```python
from build123d import *

# Parameters (mm, degrees)
SKETCH_1_W       = 99.3
SKETCH_1_H       = 96.6
SKETCH_1_R       = 1.585
EXTRUDE_1_DEPTH  = 1.5
SKETCH_2_W       = 9.8
SKETCH_2_H       = 12
EXTRUDE_2_DEPTH  = 7
SKETCH_3_R       = 3
EXTRUDE_3_DEPTH  = 9
SKETCH_4_W       = 5.1
SKETCH_4_H       = 86.4
EXTRUDE_4_DEPTH  = 8
SKETCH_5_W       = 16.4
SKETCH_5_H       = 22.2
EXTRUDE_5_DEPTH  = 13
SKETCH_6_W       = 14.42
SKETCH_6_H       = 13.5
EXTRUDE_6_DEPTH  = 6
SKETCH_7_W       = 24.3
SKETCH_7_H       = 6.4
EXTRUDE_7_DEPTH  = 2
SKETCH_8_W       = 10
SKETCH_8_H       = 10.1
EXTRUDE_8_DEPTH  = 2
SKETCH_9_W       = 9
SKETCH_9_H       = 8
EXTRUDE_9_DEPTH  = 3
SKETCH_10_W      = 13
SKETCH_10_H      = 15
EXTRUDE_10_DEPTH = 4
SKETCH_11_W      = 17
SKETCH_11_H      = 16.7
EXTRUDE_11_DEPTH = 2


with BuildPart() as part:
    # 草图1 → 凸台-拉伸1 (new body)
    with BuildSketch(Plane.XY):
        with Locations((31.77, 34.42)):
            Rectangle(SKETCH_1_W, SKETCH_1_H)
        with Locations((48.92, 64.16)):
            Circle(SKETCH_1_R, mode=Mode.SUBTRACT)
        with Locations((4.42, 64.16)):
            Circle(SKETCH_1_R, mode=Mode.SUBTRACT)
        with Locations((4.42, 4.42)):
            Circle(SKETCH_1_R, mode=Mode.SUBTRACT)
        with Locations((48.92, 4.42)):
            Circle(SKETCH_1_R, mode=Mode.SUBTRACT)
        with Locations((-9.08, 2.42)):
            Circle(SKETCH_1_R, mode=Mode.SUBTRACT)
        with Locations((72.92, -9.58)):
            Circle(SKETCH_1_R, mode=Mode.SUBTRACT)
        with Locations((72.92, 78.42)):
            Circle(SKETCH_1_R, mode=Mode.SUBTRACT)
        with Locations((-9.58, 79.42)):
            Circle(SKETCH_1_R, mode=Mode.SUBTRACT)
    extrude(amount=EXTRUDE_1_DEPTH)

    # 草图2 → 凸台-拉伸2 (add)
    with BuildSketch(Plane.XY.offset(1.5)):
        with Locations((-6.08, -7.88)):
            Rectangle(SKETCH_2_W, SKETCH_2_H)
    extrude(amount=EXTRUDE_2_DEPTH)

    # 草图3 → 凸台-拉伸3 (add)
    with BuildSketch(Plane.XY.offset(8.5)):
        with Locations((-6.18, -7.88)):
            Circle(SKETCH_3_R)
    extrude(amount=EXTRUDE_3_DEPTH)

    # 草图4 → 凸台-拉伸4 (add)
    with BuildSketch(Plane.XY.offset(1.5)):
        with Locations((78.87, 34.62)):
            Rectangle(SKETCH_4_W, SKETCH_4_H)
        with Locations((-15.33, 34.62)):
            Rectangle(SKETCH_4_W, SKETCH_4_H)
    extrude(amount=EXTRUDE_4_DEPTH)

    # 草图5 → 凸台-拉伸5 (add)
    with BuildSketch(Plane.XY.offset(1.5)):
        with Locations((61.52, 71.62)):
            Rectangle(SKETCH_5_W, SKETCH_5_H)
    extrude(amount=EXTRUDE_5_DEPTH)

    # 草图6 → 凸台-拉伸6 (add)
    with BuildSketch(Plane.XY.offset(1.5)):
        with Locations((42.11, 75.97)):
            Rectangle(SKETCH_6_W, SKETCH_6_H)
    extrude(amount=EXTRUDE_6_DEPTH)

    # 草图7 → 凸台-拉伸7 (add)
    with BuildSketch(Plane.XY.offset(1.5)):
        with Locations((19.37, 79.52)):
            Rectangle(SKETCH_7_W, SKETCH_7_H)
    extrude(amount=EXTRUDE_7_DEPTH)

    # 草图8 → 凸台-拉伸8 (add)
    with BuildSketch(Plane.XY.offset(1.5)):
        with Locations((-1.48, 76.07)):
            Rectangle(SKETCH_8_W, SKETCH_8_H)
    extrude(amount=EXTRUDE_8_DEPTH)

    # 草图9 → 凸台-拉伸9 (add)
    with BuildSketch(Plane.XY.offset(1.5)):
        with Locations((5.32, -9.88)):
            Rectangle(SKETCH_9_W, SKETCH_9_H)
    extrude(amount=EXTRUDE_9_DEPTH)

    # 草图10 → 凸台-拉伸10 (add)
    with BuildSketch(Plane.XY.offset(1.5)):
        with Locations((19.72, -6.38)):
            Rectangle(SKETCH_10_W, SKETCH_10_H)
    extrude(amount=EXTRUDE_10_DEPTH)

    # 草图11 → 凸台-拉伸11 (add)
    with BuildSketch(Plane.XY.offset(1.5)):
        with Locations((37.62, -5.53)):
            Rectangle(SKETCH_11_W, SKETCH_11_H)
    extrude(amount=EXTRUDE_11_DEPTH)


solid = part.part
```
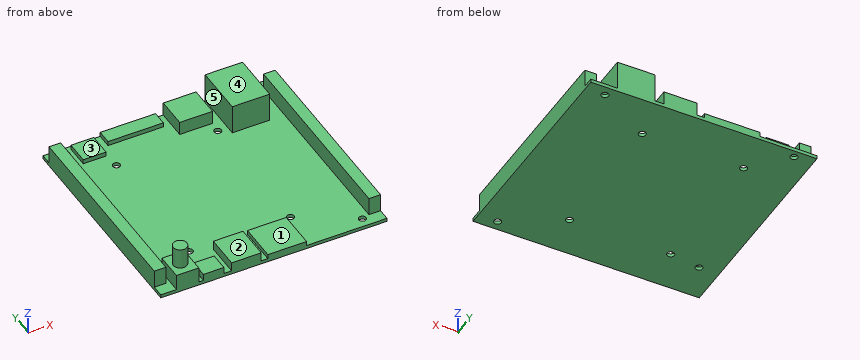
The listing builds one solid part. Answer for the finished solid, in the listing's coordinates (mm). Face numbers are marked on the shaded views. A direction names the side the tool comes from. Give positions to 0.01 mm unless a question says otherwise; leave off trailing zeros. Order: outer loops, then holes, each group sorted by start corner. A loop starts at its lowest first (then second) coordinate and runs counter-clockwise, first axis right, second up. Notation, with made-up numbers: (64, -0.5) -> (118, -0.5) arc R10 cw to (118, 12.5) -> close; hole circle Ø10 at (40.5, 41.5). An arc over 180 degrees is marked (long way). Answer as CSV lines item,"result". Start each with the question number.
Q1. A cutting plane is placed at A-A (y = 64.16). Determine the outline of the cut face in (x, z) (3 decimals).
Q2. Determine the mould class of the marked faces 4 and 5 for opening direction X: pulls with the +X half, pulls with the -X half, needs draft (parallel to the pull), parting line crosses it, or undercut.
Q3. A cutting plane is placed at D-D (x = 63). Determine the outline of the cut face in (y, z).
Q4. A cutting plane is placed at C-C (y = 27). Determine the outline of the cut face in (x, z), then the cut area to 3 significant figures.
Q5. A cutting plane is placed at B-B (z = 11.5). Determine the outline of the cut face in (x, y), then the cut area to 3 significant figures.
Q6. Which of the six approach directions +Z, -Z, +X, -X, +Y, -Y give full straight-line access (tool end or side, diameter ignored) to the marked faces 1, 2 and 3?
Q7. Given pin 1 (4 mm diameter, centred on x = 79, z = 5, fed in from -Y); pin 2 (2.5 mm diameter, centred on x = 78.5, z = 5.5, fed in from +Y); pin 3 (7 mm diameter, centred on x = 14.5, y = 79.5, fed in from +Z), each flat-ended and moving along its own axis, determine where each tip first touches the part or whether it passes through.
Q8. Find the intervals of material crossed by L1, parallel to Y at x = 48.92, z = 0.8 (3 decimals); L2, parallel to Y at x = -9.58, z = 0.85 (3 decimals); L3, parallel to X at y = 64.16, z = 0.75 (3 decimals), in increasing order.
Results found:
1,outline,"(-17.88, 0) -> (2.835, 0) -> (2.835, 1.5) -> (-12.78, 1.5) -> (-12.78, 9.5) -> (-17.88, 9.5) -> close; (6.005, 0) -> (47.335, 0) -> (47.335, 1.5) -> (6.005, 1.5) -> close; (50.505, 0) -> (81.42, 0) -> (81.42, 9.5) -> (76.32, 9.5) -> (76.32, 1.5) -> (69.72, 1.5) -> (69.72, 14.5) -> (53.32, 14.5) -> (53.32, 1.5) -> (50.505, 1.5) -> close"
2,face 4,"needs draft"
2,face 5,"undercut"
3,outline,"(-13.88, 0) -> (82.72, 0) -> (82.72, 14.5) -> (60.52, 14.5) -> (60.52, 1.5) -> (-13.88, 1.5) -> close"
4,outline,"(-17.88, 0) -> (81.42, 0) -> (81.42, 9.5) -> (76.32, 9.5) -> (76.32, 1.5) -> (-12.78, 1.5) -> (-12.78, 9.5) -> (-17.88, 9.5) -> close"
4,area,"231 mm2"
5,outline,"circle Ø6 at (-6.18, -7.88); (53.32, 60.52) -> (69.72, 60.52) -> (69.72, 82.72) -> (53.32, 82.72) -> close"
5,area,"392 mm2"
6,face 1,"+Z, -Y"
6,face 2,"+Z, +Y, -Y"
6,face 3,"+Z, +Y"
7,pin 1,"y = -8.58"
7,pin 2,"y = 77.82"
7,pin 3,"z = 3.5"
8,L1,"-13.88 to 2.835, 6.005 to 62.575, 65.745 to 82.72"
8,L2,"-13.88 to 0.916, 3.924 to 77.835, 81.005 to 82.72"
8,L3,"-17.88 to 2.835, 6.005 to 47.335, 50.505 to 81.42"
